Model file for the job. Use its own axes, mm. A direction names the side the tool comes from. Round coordinates to 2 decimals unless told otherwise and drop trailing zeros. Order: outer loops, then holes, each group sorted by start corner. A loop starts at its lowest first (then second) coordinate and runs counter-clockwise, first axis right, second up. Notation, with made-up numbers: (64, 29) - (119, 29) arc R18 ccw to (119, 64) - close; hole circle Ø10 at (13, 31). An arc over 180 degrees is marked (long way). Answer as CSV lines item,"result". Start each with the question number.
1. Band-saw the part on C-C on x = -8.5. List the corners of the cut face in (y, z), then the cut area to 3 significant figures.
2. Pull direction Y, two halves, no side cores. Call faces 4 (the face through (-12, 10, -57)), 5 (the face through (0, 20, 1)), 6 (the face through (-1, 1, 1)), 7 (the face through (-1, 19, 1)): released by +Y, released by -Y, zero draft, split by the parting line, or undercut.
3. Wall check: line 1 along Y through (x, z) = (2.2, 46); line 2 along Y through (x, z) = (1.5, 9); line 3 along Y through (x, z) = (-0.75, 26). Give the ranges that are in metal, low to high. Write a range as [from, to].
4. Band-saw the part on A-A on z = 24.5. List the corners of the cut face in (x, y).
5. Band-saw the part on B-B on y = 4.75. List the corners of the cut face in (x, z).
6. Pin check, flat tips, straight feed: pin 1 Ø1.5 at (y, z) = (2, 22) entering from -X; pin 2 Ø1 at (x, y) = (-8.5, -0.5) entering from +Z; pin 3 Ø2 at (x, z) = (1, -40) entering from -Y. Stop position of each tip, or through.
7. 3-axis set-ups, long thin cutter, end or side, ignore diameter. For faces 1 (the face through (0, 0, 1)), 2 (the face through (0.5, 10, 1)), 3 (the face through (-4, 25, -57)): which of +Z, -Z, +X, -X, +Y, -Y reach the whole face in a straight line?
Autodesk Inventor part; units mm, degrees
ref_plane "Work Plane2" through (0, 10, 0) normal (0, 1, 0) x (-1, 0, 0)
ref_plane "YZ Plane" through (0, 0, 0) normal (1, 0, 0) x (0, 1, 0)
ref_plane "XY Plane" through (0, 0, 0) normal (0, 0, 1) x (1, 0, 0)
sketch "Sketch1" plane through (0, 0, 0) normal (0, 1, 0) x (-1, 0, 0)
  line L0 (-3, 50) -> (3, 50)
  line L1 (3, 50) -> (3, -50)
  line L2 (3, -50) -> (-3, -50)
  line L3 (-3, -50) -> (-3, 50)
  line L4 (-3, 50) -> (3, -50) construction
  line L5 (3, 50) -> (-3, -50) construction
  point P0 (0, 0)
  dimension "d123" = 6
  dimension "d124" = 100
extrude "Extrusion1" add sketch "Sketch1" along normal blind 20
sketch "Sketch2" plane through (0, 0, -50) normal (0, 0, -1) x (-1, 0, 0)
  line L0 (-3, 25) -> (12, 25)
  line L1 (12, 25) -> (12, -5)
  line L2 (12, -5) -> (-3, -5)
  line L3 (-3, -5) -> (-3, 25)
  line L4 (3, 0) -> (3, 20)
  line L5 (-3, 25) -> (12, -5) construction
  line L6 (12, 25) -> (-3, -5) construction
  line L7 (-3, 0) -> (-3, 20)
  line L8 (-3, 20) -> (3, 20)
  line L9 (0, 20) -> (0, 0) construction
  circle A0 centre (-1.5, 18.5) radius 0.5
  circle A1 centre (-1.5, 10) radius 0.5
  line L10 (-3, 10) -> (3, 10) construction
  circle A2 centre (-1.5, 1.5) radius 0.5
  line L11 (-0.5, 1) -> (-0.5, 19)
  dimension "d125" = 15
  dimension "d126" = 30
  dimension "d127" = 5
  dimension "d128" = 9
  dimension "d129" = 1
  dimension "d130" = 1.5
  dimension "d131" = 1.5
  dimension "d132" = 1
  dimension "d133" = 1.5
  dimension "d134" = 10
extrude "Extrusion21" add sketch "Sketch2" along normal blind 15 contours L0 L1 L2 L3 | A0 | A1 | A2
extrude "Extrusion22" cut sketch "Sketch2" along normal blind 15 and the other way blind 100 contours A0 | A1 | A2
sketch "Sketch15" plane through (-3, 0, 50) normal (0, 0, 1) x (1, 0, 0)
  line L0 (3.5, 1) -> (-3.5, 1)
  line L1 (-3.5, 1) -> (-3.5, 19)
  line L2 (-3.5, 19) -> (3.5, 19)
  line L3 (3.5, 19) -> (3.5, 1)
  line L4 (0, 0) -> (0, 20)
  line L5 (3.5, 1) -> (-3.5, 19) construction
  line L6 (-3.5, 1) -> (3.5, 19) construction
  point P0 (3, 0)
  point P1 (0, 10)
  dimension "d145" = 7
  dimension "d146" = 18
extrude "Extrusion24" cut sketch "Sketch15" against normal blind 100
sketch "Sketch16" plane through (3, 0, 50) normal (1, 0, 0) x (0, 0, -1)
  line L0 (100, 20) -> (0, 20) construction
  line L1 (4, 20) -> (4, 0) construction
  line L2 (100, 0) -> (0, 0) construction
  line L3 (0, 0) -> (0, 20) construction
  circle A0 centre (4, 18.5) radius 0.5
  line L4 (0, 10.5) -> (115, 10.5)
  circle A1 centre (4, 10.5) radius 0.5
  circle A2 centre (4, 1.5) radius 0.5
  point P0 (50, 0)
  dimension "d149" = 4
  dimension "d150" = 1
  dimension "d151" = 1
  dimension "d152" = 1.5
  dimension "d154" = 1
  dimension "d155" = 1.5
extrude "Extrusion25" cut sketch "Sketch16" against normal blind 1.5
fillet "Fillet4" radius 3 2 edges at (-3, 19.5, 50) (-3, 0.5, 50)
sketch "Sketch6" plane through (0, 10, 0) normal (0, 1, 0) x (-1, 0, 0)
  line L0 (21.0864, 109.726) -> (-9.863, 109.726)
  line L1 (-9.863, 109.726) -> (-9.863, -3.5286)
  line L2 (-9.863, -3.5286) -> (21.0864, -3.5286)
  line L3 (21.0864, -3.5286) -> (21.0864, 109.726)
  point P0 (0, 0)
  dimension "d36" = 113.2546
  dimension "d37" = 30.9494
properties part number "3D_print_actuator_cable_driven"
Reply:
1,outline,"(-5, -65) - (25, -65) - (25, -50) - (-5, -50) - close"
1,area,"450 mm2"
2,face 4,"zero draft"
2,face 5,"released by +Y"
2,face 6,"undercut"
2,face 7,"undercut"
3,line 1,"y = [0, 1], [2, 10], [11, 18], [19, 20]"
3,line 2,"y = [0, 1], [2, 9.5], [10.5, 18], [19, 20]"
3,line 3,"y = [0, 1], [19, 20]"
4,outline,"(-3, 0) - (3, 0) - (3, 20) - (-3, 20) - (-3, 19) - (0.5, 19) - (0.5, 1) - (-3, 1) - close; hole circle Ø1 at (1.5, 1.5); hole circle Ø1 at (1.5, 10); hole circle Ø1 at (1.5, 18.5)"
5,outline,"(-12, -65) - (3, -65) - (3, 50) - (0.5, 50) - (0.5, -50) - (-12, -50) - close"
6,pin 1,"stops at x = 0.5"
6,pin 2,"stops at z = -50"
6,pin 3,"stops at y = 0"
7,face 1,"+Z, +X, -X, -Y"
7,face 2,"+Z, -X"
7,face 3,"+Z, -Z, +X, -X, +Y"
